from build123d import *

# Parameters (mm, degrees)
SKETCH2_W                 = 68.7
SKETCH2_H                 = 53.6
PCB_DEPTH                 = 1.5
BARREL_START              = 1.5
SKETCH3_W                 = 14.25
SKETCH3_H                 = 9
BARREL_JACK_DEPTH         = 11.1
HWSERIAL_START            = 1.5
SKETCH4_W                 = 16.4
SKETCH4_H                 = 12.1
HWSERIAL_PORT_DEPTH       = 11
BOSS_EXTRUDE4_START       = 1.5
SKETCH5_W                 = 47.73
SKETCH5_H                 = 2.4
SKETCH5_W_2               = 38.7
BOSS_EXTRUDE4_DEPTH       = 8.67
F_3_0MM_DOWEL_HOLE1_D     = 3
F_3_0MM_DOWEL_HOLE1_DEPTH = 7.5
F_3_0MM_DOWEL_HOLE1_TIP   = 0.901290929


with BuildPart() as part:
    # Sketch2 → PCB (new body)
    with BuildSketch(Plane(origin=(0, 0, 0), x_dir=(1, 0, 0), z_dir=(0, 1, 0))):
        with Locations((34.35, 26.8)):
            Rectangle(SKETCH2_W, SKETCH2_H)
    extrude(amount=PCB_DEPTH)

    # Sketch3 → Barrel Jack (add)
    with BuildSketch(Plane(origin=(0, 0, 0), x_dir=(1, 0, 0), z_dir=(0, 1, 0)).offset(BARREL_START)):
        with Locations((3.725, 8.75)):
            Rectangle(SKETCH3_W, SKETCH3_H)
    extrude(amount=BARREL_JACK_DEPTH)

    # Sketch4 → HWSerial Port (add)
    with BuildSketch(Plane(origin=(0, 0, 0), x_dir=(1, 0, 0), z_dir=(0, 1, 0)).offset(HWSERIAL_START)):
        with Locations((1.4, 39.05)):
            Rectangle(SKETCH4_W, SKETCH4_H)
    extrude(amount=HWSERIAL_PORT_DEPTH)

    # Sketch5 → Boss-Extrude4 (add)
    with BuildSketch(Plane(origin=(0, 0, 0), x_dir=(1, 0, 0), z_dir=(0, 1, 0)).offset(BOSS_EXTRUDE4_START)):
        with Locations((40.865, 50.2)):
            Rectangle(SKETCH5_W, SKETCH5_H)
        with Locations((45.35, 2.9)):
            Rectangle(SKETCH5_W_2, SKETCH5_H)
    extrude(amount=BOSS_EXTRUDE4_DEPTH)

    # Ø3.0mm Dowel Hole1
    with Locations(Plane(origin=(0, 1.5, 0), x_dir=(1, 0, 0), z_dir=(0, 1, 0))):
        with Locations((15, 51.1), (14, 2.5), (66, 7.5), (66.2, 33.5)):
            Hole(F_3_0MM_DOWEL_HOLE1_D / 2, depth=F_3_0MM_DOWEL_HOLE1_DEPTH)
            with Locations((0, 0, -(F_3_0MM_DOWEL_HOLE1_DEPTH + F_3_0MM_DOWEL_HOLE1_TIP / 2))):  # 118° drill point
                Cone(0, F_3_0MM_DOWEL_HOLE1_D / 2, F_3_0MM_DOWEL_HOLE1_TIP, mode=Mode.SUBTRACT)


solid = part.part
Geometry: final body of the model. Coordinates: model frame, mm. A direction names the side the tool comes from. Give positions to 0.01 mm unless a question says otherwise; leave off trailing zeros. Loops run counter-clockwise (first coordinate to the right, second up) from the corner with the lowest first, then second, coordinate; pieces in that order, holes last. Notation, with made-up numbers: M -2.5,21 L 7.5,21 A20 ccw 7.5,42 Z; hole C 54,80 d6. An arc over 180 degrees is marked long. Put each result on its own line as item: value. Start each with the question number.
1) Ray query, line 1 along Z through (x, y) = (66.2, 0.5); line 2 along Z through (x, y) = (1.5, 3); line 3 along X through (y, z) = (0.95, -33.5). Return the intervals inside material, ascending.
2) Cut plane C-C (z = -2.5). Output: boundary loops of the cut face in (x, y).
3) Contact query for flat-ended pins moving along their axis: pin 1 (3.5 mm diameter, centred on x = 4.5, y = 6, fed in from -Z); pin 2 (1.5 mm diameter, centred on x = 19, y = 7.5, fed in from +Z); pin 3 (2.5 mm diameter, centred on y = 4.5, z = -50, fed in from -X); pin 4 (2.5 mm diameter, centred on x = 14, z = -2.5, fed in from +Y). Output: stop coordinate, or through.
4) Access query for faces 1 (the flat face through (9.6, 7, -39)), 2 (the flat face through (1, 7, -33)), 3 (the flat face through (4, 7, -4.25)), 4 (the flat face through (-3, 1.5, -39)). Directions: +Z, -Z, +X, -X, +Y, -Y. A direction counts if a zero-diameter tool reaches every point of the face in a straight line with its end or side. Return the directions, or none.
5) Cut plane D-D (x = 28). Output: boundary loops of the cut face in (y, z).
6) Pull-direction query (Z, two-part tool) for faces 5 (the cylindrical face through (65.51, 0.74, -32.17)), 6 (the flat face through (1, 7, -45.1)), 7 (the flat face through (-3.4, 7, -9)); classes: pulls with the +Z half, pulls with the -Z half, needs draft (parallel to the pull), parting line crosses it, or undercut.
7) Cut plane B-B (x = -2). Output: boundary loops of the cut face in (y, z).
8) Cut plane A-A (y = 11.5). Output: boundary loops of the cut face in (x, z).
Verdict:
1. line 1: -53.6 to -35, -32 to -8.99, -6.01 to 0
1. line 2: -45.1 to -33, -13.25 to -4.25
1. line 3: 0 to 64.7, 67.7 to 68.7
2. outline: M 0,0 L 12.5,0 L 12.5,1.5 L 0,1.5 Z; M 15.5,0 L 68.7,0 L 68.7,1.5 L 64.7,1.5 L 64.7,10.17 L 26,10.17 L 26,1.5 L 15.5,1.5 Z
3. pin 1: z = -45.1
3. pin 2: z = -49
3. pin 3: x = 17
3. pin 4: through
4. face 1: -Z, +X, +Y
4. face 2: +X, -X, +Y
4. face 3: +Z, +X, -X, +Y
4. face 4: +Z, -Z, -X, -Y
5. outline: M 0,-53.6 L 1.5,-53.6 L 1.5,-51.4 L 10.17,-51.4 L 10.17,-49 L 1.5,-49 L 1.5,-4.1 L 10.17,-4.1 L 10.17,-1.7 L 1.5,-1.7 L 1.5,0 L 0,0 Z
6. face 5: undercut
6. face 6: pulls with the -Z half
6. face 7: needs draft
7. outline: M 1.5,-45.1 L 12.5,-45.1 L 12.5,-33 L 1.5,-33 Z; M 1.5,-13.25 L 12.6,-13.25 L 12.6,-4.25 L 1.5,-4.25 Z
8. outline: M -6.8,-45.1 L 9.6,-45.1 L 9.6,-33 L -6.8,-33 Z; M -3.4,-13.25 L 10.85,-13.25 L 10.85,-4.25 L -3.4,-4.25 Z
